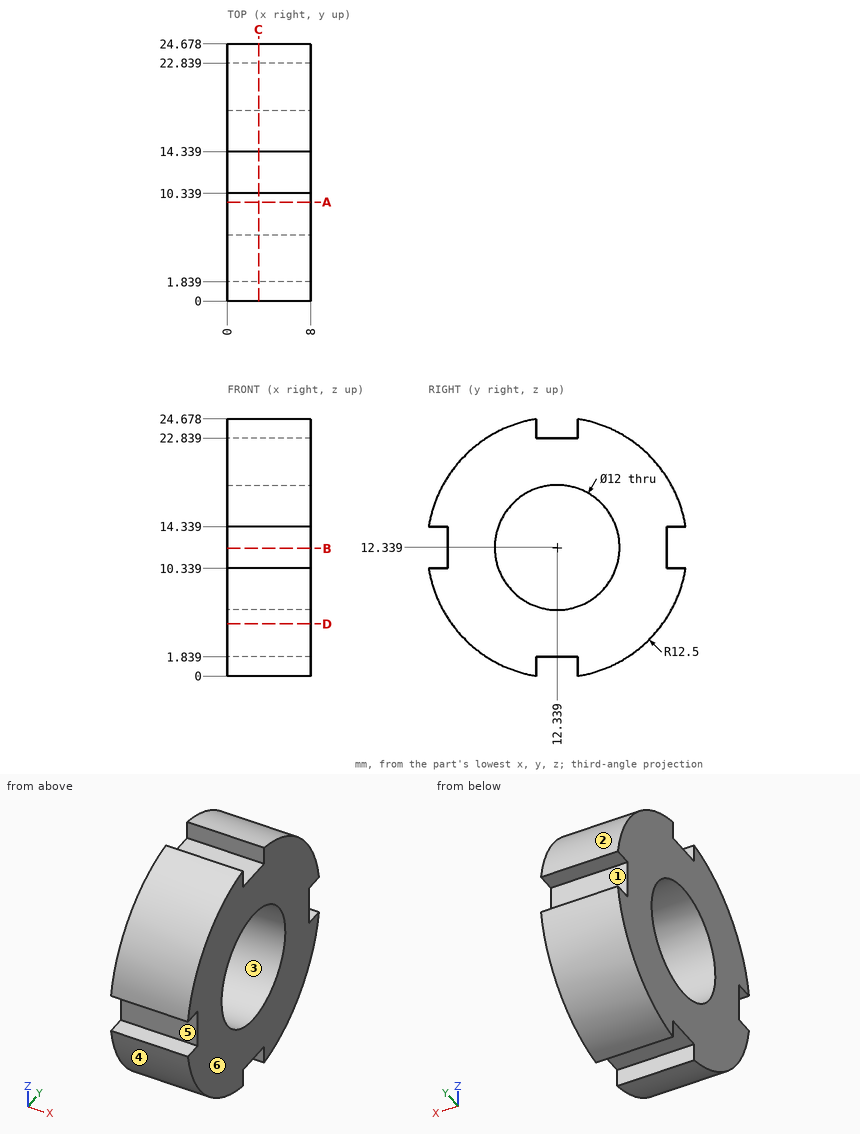
Here's the drawing with two shaded views (mm, measured from the low corner). I have some questions. A direction names the side the tool comes from. Give positions to 0.01 mm unless a question says otherwise; leave off trailing zeros. Write each loop counter-clockwise with the first axis right and the second up, starting at its lowest first coordinate (ties: lowest second). Pieces come first, ordered by that corner, then holes. Notation, with made-up numbers: (49.25, -36.75) -> (69.25, -36.75) arc R14 cw to (69.25, -23.75) -> close; hole circle Ø4 at (30.25, 26.25). An arc over 180 degrees is marked (long way). Use one line per item in the form item = value.
1) Suppose I cut it at C-C (x = 3). Please give me the cut outline in (y, z).
Verdict:
outline = (0, 10.34) arc R12.5 ccw to (10.34, 0) -> (10.34, 1.84) -> (14.34, 1.84) -> (14.34, 0) arc R12.5 ccw to (24.68, 10.34) -> (22.84, 10.34) -> (22.84, 14.34) -> (24.68, 14.34) arc R12.5 ccw to (14.34, 24.68) -> (14.34, 22.84) -> (10.34, 22.84) -> (10.34, 24.68) arc R12.5 ccw to (0, 14.34) -> (1.84, 14.34) -> (1.84, 10.34) -> close; hole circle Ø12 at (12.34, 12.34)
2) Suppose I cut it at A-A (y = 9.5). Please give me the cut outline in (x, z).
Verdict:
outline = (0, 0.17) -> (8, 0.17) -> (8, 7.05) -> (0, 7.05) -> close; (0, 17.62) -> (8, 17.62) -> (8, 24.51) -> (0, 24.51) -> close
3) Suppose I cut it at D-D (z = 5). Please give me the cut outline in (x, y), and give its area (3 significant figures).
Verdict:
outline = (0, 2.22) -> (8, 2.22) -> (8, 22.46) -> (0, 22.46) -> close
area = 162 mm2
4) Suppose I cut it at B-B (z = 12.25). Please give me the cut outline in (x, y).
Verdict:
outline = (0, 1.84) -> (8, 1.84) -> (8, 6.34) -> (0, 6.34) -> close; (0, 18.34) -> (8, 18.34) -> (8, 22.84) -> (0, 22.84) -> close
5) We'd pull the mould along Z, two halves only. Please class the marked faces 3, 4, 5 and 6: +Z half, -Z half, draft (parallel to the pull), parting line (faces both ways), or undercut.
Verdict:
face_3 = undercut
face_4 = -Z half
face_5 = undercut
face_6 = draft
6) On a 3-axis mill with a long thin cutter (end or side, diameter ignored), from which of +Z, -Z, +X, -X, +Y, -Y can I reach the whole of each face in a straight line? I mean the marked faces 1 and 2. Say none if no direction works.
Verdict:
face_1 = +X, -X, +Y
face_2 = +Z, +X, -X, +Y
7) If I drill on L1, parallel to Z at x = 7.5, y = 11.5; L2, parallel to Y at x = 3.75, z = 9.25 (1 decimal); L3, parallel to Z at x = 5.5, y = 17.75, over which ranges is the centre line in solid material (lowest first)? Write a range as [from, to].
Verdict:
L1 = [1.84, 6.4], [18.28, 22.84]
L2 = [0.2, 7.2], [17.5, 24.5]
L3 = [1.07, 9.75], [14.93, 23.61]
8) I'm going to push flat-ended pins straight in: pin 1 (3 mm diameter, centred on x = 4, y = 8.5, fed in from -Z); pin 2 (1.5 mm diameter, centred on x = 2, y = 1.5, fed in from -Z); pin 3 (1.5 mm diameter, centred on x = 3.5, y = 0.5, fed in from +Z); pin 4 (4 mm diameter, centred on x = 5, z = 12.5, fed in from -Y). Where does each tip first touch, or does it pass through?
Verdict:
pin_1 = 0.06
pin_2 = 4.96
pin_3 = 18.11
pin_4 = 0
